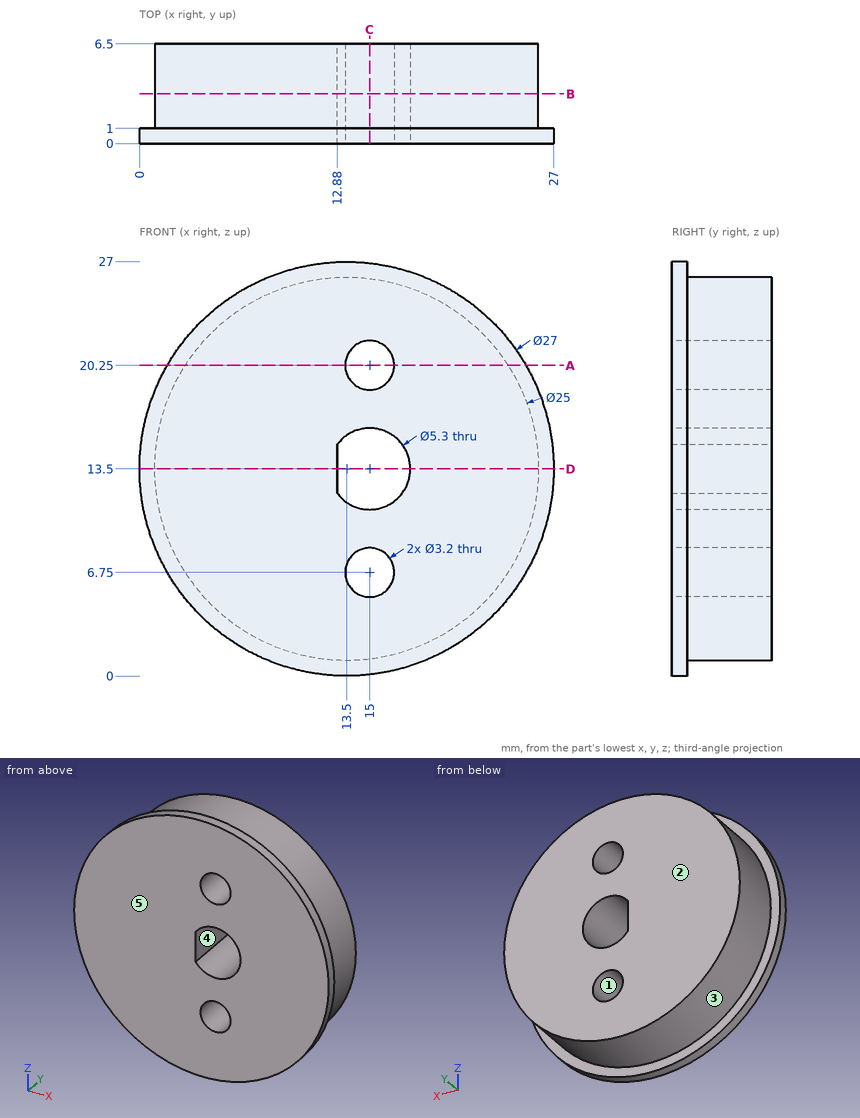
Check sheet for the drawn part. Datum: minimum x, y, z corner. Units: mm. A direction names the side the tool comes from. Round coordinates to 2 decimals unless told otherwise and drop trailing zeros. Order: outer loops, then holes, each group sorted by start corner. A loop starts at its lowest first (then second) coordinate and runs counter-clockwise, first axis right, second up. Notation, with made-up numbers: (81, 1) - (107, 1) arc R31 ccw to (107, 38) - close; hole circle Ø9 at (-9, 85.5). An arc over 180 degrees is marked (long way). Use a Markdown table: item, result. Add a question column.
(1) Depth check by flat-ended pin: pin 1 (1 mm diameter, centred on y = 1, z = 14.5, fed in from +X); pin 2 (1.6 mm diameter, centred on y = 2, z = 13, fed in from +X); pin 3 (2 mm diameter, centred on x = 11.5, y = 2.5, fed in from +Z). Enter the tip coordinate at first touch or a pass-through.
(2) Sectioned sample at C-C, the plane x = 15. Enter the section's corners in (y, z).
(3) Sectioned sample at A-A, the plane z = 20.25. Enter the section's corners in (x, y).
(4) Material ranges on line 1 along X through (y, z) = (5.25, 13.5); line 2 along Z through (x, y) = (15, 3.5); line 3 along Y through (x, z) = (6.25, 24), recorded low to high. Write a range as [from, to].
(5) Release check for a two-part mould opening along Z. For the marked faces 1, 2 and 3 record: pulls with the +Z half, pulls with the -Z half, needs draft (parallel to the pull), parting line crosses it, or undercut.
(6) Sectioned sample at B-B, the plane y = 3.25. Enter the section's corners in (x, z), and give its area (3 significant figures).
(7) Tool access check on the marked faces 4 and 5. Record the directions out of +Z, -Z, +X, -X, +Y, -Y that give a thin tool (end or side, any length) a straight path to the whole face; none if there is none.
(8) Sectioned sample at D-D, the plane z = 13.5. Enter the section's corners in (x, y), and give its area (3 significant figures).
Answers below:
| question | item | result |
|---|---|---|
| 1 | pin 1 | x = 26.99 |
| 1 | pin 2 | x = 26 |
| 1 | pin 3 | z = 25.96 |
| 2 | outline | (0, 0.08) - (1, 0.08) - (1, 1.09) - (6.5, 1.09) - (6.5, 5.15) - (0, 5.15) - close; (0, 8.35) - (6.5, 8.35) - (6.5, 10.85) - (0, 10.85) - close; (0, 16.15) - (6.5, 16.15) - (6.5, 18.65) - (0, 18.65) - close; (0, 21.85) - (6.5, 21.85) - (6.5, 25.91) - (1, 25.91) - (1, 26.92) - (0, 26.92) - close |
| 3 | outline | (1.81, 0) - (13.4, 0) - (13.4, 6.5) - (2.98, 6.5) - (2.98, 1) - (1.81, 1) - close; (16.6, 0) - (25.19, 0) - (25.19, 1) - (24.02, 1) - (24.02, 6.5) - (16.6, 6.5) - close |
| 4 | line 1 | [1, 12.88], [17.65, 26] |
| 4 | line 2 | [1.09, 5.15], [8.35, 10.85], [16.15, 18.65], [21.85, 25.91] |
| 4 | line 3 | [0, 1] |
| 5 | face 1 | undercut |
| 5 | face 2 | needs draft |
| 5 | face 3 | parting line crosses it |
| 6 | outline | circle Ø25 at (13.5, 13.5); hole (12.88, 11.91) arc R2.65 ccw (long way) to (12.88, 15.09) - close; hole circle Ø3.2 at (15, 6.75); hole circle Ø3.2 at (15, 20.25) |
| 6 | area | 454 mm² |
| 7 | face 4 | +Y, -Y |
| 7 | face 5 | +Z, -Z, +X, -X, -Y |
| 8 | outline | (0, 0) - (12.88, 0) - (12.88, 6.5) - (1, 6.5) - (1, 1) - (0, 1) - close; (17.65, 0) - (27, 0) - (27, 1) - (26, 1) - (26, 6.5) - (17.65, 6.5) - close |
| 8 | area | 133 mm² |
